Here's how the part is built. I have some questions about the finished solid (model axes, mm). A direction names the side the tool comes from. Give positions to 0.01 mm unless a question says otherwise; leave off trailing zeros. Order: outer loops, then holes, each group sorted by start corner. A loop starts at its lowest first (then second) coordinate and runs counter-clockwise, first axis right, second up.
from build123d import *

# Parameters (mm, degrees)
SKETCH1_W           = 6.35
SKETCH1_H           = 6.35
BOSS_EXTRUDE1_DEPTH = 10.16
CUT_EXTRUDE1_DEPTH  = 6.35


with BuildPart() as part:
    # Sketch1 → Boss-Extrude1 (new body, symmetric)
    with BuildSketch(Plane(origin=(0, 0, 0), x_dir=(1, 0, 0), z_dir=(0, 1, 0))):
        Rectangle(SKETCH1_W, SKETCH1_H)
    extrude(amount=BOSS_EXTRUDE1_DEPTH, both=True)

    # Sketch2 → Cut-Extrude1 (cut)
    with BuildSketch(Plane(origin=(3.175, 0, 0), x_dir=(0, 0, -1), z_dir=(1, 0, 0))):
        with BuildLine():
            Line((-3.175, 0.254), (-3.175, -0.254))
            Line((-3.175, -0.254), (-2.667, -0.254))
            Line((-2.667, -0.254), (-1.6002, -1.5875))
            ThreePointArc((-1.6002, -1.5875), (-0.0127, 0), (-1.6002, 1.5875))
            Line((-1.6002, 1.5875), (-2.667, 0.254))
            Line((-2.667, 0.254), (-3.175, 0.254))
        make_face()
    cut_extrude1 = extrude(amount=-CUT_EXTRUDE1_DEPTH, mode=Mode.SUBTRACT)

    # Mirror1: Cut-Extrude1 across plane
    add(cut_extrude1.mirror(Plane.XY), mode=Mode.SUBTRACT)


solid = part.part
Q1. If we section it at B-B on z = -0.75: List the corners of the cut face in (x, y) for me (3 decimals).
Filled sheet:
outline: (-3.175, -10.16) - (3.175, -10.16) - (3.175, -1.341) - (-3.175, -1.341) - close; (-3.175, 1.341) - (3.175, 1.341) - (3.175, 10.16) - (-3.175, 10.16) - close
Q2. Thinking about a two-plate mould opening in Y: for faces 3 (the face through (0.04, -0.91, 2.14)), 4 (the face through (0, -10.16, 0)), 5 (the face through (0.044, -0.576, -0.121)), 6 (the face through (0, -5, 3.175)), which applies, released by +Y, released by -Y, zero draft, split by the parting line, or undercut?
Filled sheet:
face 3: undercut
face 4: released by -Y
face 5: undercut
face 6: zero draft
Q3. I need wall thicknesses on L1, parallel to Y at x = 1.75, z = 1.5; L2, parallel to Z at x = 0.5, y = 1 (3 decimals); L3, parallel to Y at x = -3, z = -1.25. Which ranges of each line are inside material? Lowest first, please.
Filled sheet:
L1: y = -10.16 to -1.58, 1.58 to 10.16
L2: z = -3.175 to -2.07, -0.367 to 0.367, 2.07 to 3.175
L3: y = -10.16 to -1.55, 1.55 to 10.16
Q4. For faces 1 (the face through (0.04, -0.91, -2.14)), 2 (the face through (0, 10.16, 0)), which set-ups out of +Z, -Z, +X, -X, +Y, -Y let a thin tool reach every point of the face, with its end or its side?
Filled sheet:
face 1: +X, -X
face 2: +Z, -Z, +X, -X, +Y
Q5. If we section it at D-D on z = -2: List the corners of the cut face in (x, y) for me (3 decimals).
Filled sheet:
outline: (-3.175, -10.16) - (3.175, -10.16) - (3.175, -1.088) - (-3.175, -1.088) - close; (-3.175, 1.088) - (3.175, 1.088) - (3.175, 10.16) - (-3.175, 10.16) - close
Q6. If we section it at A-A on x = 1: List the corners of the cut face in (y, z) for me (1 decimal).
Filled sheet:
outline: (-10.2, -3.2) - (-0.3, -3.2) - (-0.3, -2.7) - (-1.6, -1.6) arc R1.6 cw to (1.6, -1.6) - (0.3, -2.7) - (0.3, -3.2) - (10.2, -3.2) - (10.2, 3.2) - (0.3, 3.2) - (0.3, 2.7) - (1.6, 1.6) arc R1.6 cw to (-1.6, 1.6) - (-0.3, 2.7) - (-0.3, 3.2) - (-10.2, 3.2) - close
